Check sheet for the modelled part. Datum: model origin and axes. Units: mm. Coordinates: 2 decimals unless noted, no trailing zeros. Loops run counter-clockwise (first coordinate to the right, second up) from the corner with the lowest first, then second, coordinate; pieces in that order, holes last.
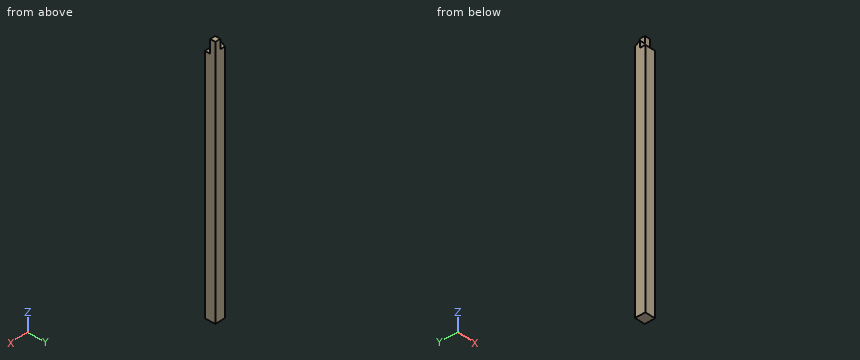
```python
from build123d import *

# Parameters (mm, degrees)
F0_W          = 100
F0_H          = 100
F1_DEPTH      = 2400
F2_W          = 50
F2_H          = 125
F3_DEPTH      = 50
F3_DEPTH_BACK = 50
F5_DEPTH      = 50


with BuildPart() as f1:
    # F0 (on Top) → F1 (new body)
    with BuildSketch(Plane.XY):
        Rectangle(F0_W, F0_H)
    extrude(amount=F1_DEPTH)

    # F2 (on Right) → F3 (cut, two sides)
    with BuildSketch(Plane.YZ) as f3_sk:
        with Locations((-25, 2337.5)):
            Rectangle(F2_W, F2_H)
    extrude(amount=-F3_DEPTH, mode=Mode.SUBTRACT)
    extrude(f3_sk.sketch, amount=F3_DEPTH_BACK, mode=Mode.SUBTRACT)

    # F4 (on face) → F5 (cut)
    with BuildSketch(Plane(origin=(-50, 0, 0), x_dir=(0, -1, 0), z_dir=(-1, 0, 0))):
        Polygon((0, 2400), (-50, 2400), (-50, 2310.246), (0, 2335.246), align=None)
    extrude(amount=-F5_DEPTH, mode=Mode.SUBTRACT)


solid = f1.part
```
1) Section check B-B on y = -35. Enter the section's corners in (x, z).
Answer sheet:
outline: (-50, 0) - (50, 0) - (50, 2275) - (-50, 2275) - close
2) Scan lines: line 1 (Z direction, x = 27, y = -36); line 2 (Z direction, x = -14.5, y = 37.5). Record each from-to range of solid material in increasing order.
Answer sheet:
line 1: z = 0 to 2275
line 2: z = 0 to 2316.5
3) Section check A-A on x = 27.5. Enter the section's corners in (y, z).
Answer sheet:
outline: (-50, 0) - (50, 0) - (50, 2400) - (0, 2400) - (0, 2275) - (-50, 2275) - close
4) Depth check by flat-ended pin: pin 1 (2 mm diameter, centred on x = -31, y = -19, fed in from +Z). Enter the tip coordinate at first touch or a pass-through.
Answer sheet:
pin 1: stops at z = 2275
